CAD build for the part. Positions are in the model's coordinates, mm. Coordinates: 2 decimals unless noted, no trailing zeros. Order: outer loops, then holes, each group sorted by start corner. A loop starts at its lowest first (then second) coordinate and runs counter-clockwise, first axis right, second up. Notation, with made-up numbers: M 56.5,-14 L 103.5,-14 A30 cw 103.5,11 Z; hole C 10,9 d8. An arc over 180 degrees is marked long. Write item = value, one per line.
from build123d import *

# Parameters (mm, degrees)
SKETCH1_W           = 71.428571428
SKETCH1_H           = 3.175
SKETCH1_W_2         = 20
SKETCH1_W_3         = 18.5
BOSS_EXTRUDE1_DEPTH = 3.175


with BuildPart() as part:
    # Sketch1 → Boss-Extrude1 (new body)
    with BuildSketch(Plane.XY):
        Polygon((0, 0), (0, 132.75), (0, 252.75), (278.222222222, 252.75), (313, 252.75), (313, 228.115), (313, 132.75), (357.142857143, 132.75), (357.142857143, 129.575), (428.571428571, 129.575), (428.571428571, 132.75), (500, 132.75), (500, 0), (428.571428571, 0), (428.571428571, 3.175), (357.142857143, 3.175), (357.142857143, 0), (285.714285714, 0), (285.714285714, 3.175), (214.285714286, 3.175), (214.285714286, 0), (142.857142857, 0), (142.857142857, 3.175), (71.428571429, 3.175), (71.428571429, 0), align=None)
        with Locations((107.142857143, 131.1625)):
            Rectangle(SKETCH1_W, SKETCH1_H, mode=Mode.SUBTRACT)
        with Locations((250, 131.1625)):
            Rectangle(SKETCH1_W, SKETCH1_H, mode=Mode.SUBTRACT)
        with Locations((14, 60.0875)):
            Rectangle(SKETCH1_W_2, SKETCH1_H, mode=Mode.SUBTRACT)
        with Locations((14, 72.6625)):
            Rectangle(SKETCH1_W_2, SKETCH1_H, mode=Mode.SUBTRACT)
        with Locations((472.25, 33.2875)):
            Rectangle(SKETCH1_W_3, SKETCH1_H, mode=Mode.SUBTRACT)
        with Locations((472.25, 99.4625)):
            Rectangle(SKETCH1_W_3, SKETCH1_H, mode=Mode.SUBTRACT)
    extrude(amount=BOSS_EXTRUDE1_DEPTH)


solid = part.part
(1) Pin check, flat tips, straight feed: pin 1 Ø1.6 at (y, z) = (131, 1) entering from -X; pin 2 Ø1 at (x, z) = (472, 1) entering from +Y; pin 3 Ø1 at (x, z) = (260, 2) entering from -Y (3 decimals). Stop position of each tip, or through.
Evaluation:
pin_1 = 0
pin_2 = 132.75
pin_3 = 3.175
(2) Slice it at C-C, the plane x = 375. Write the cut outline in (y, z) (3 decimals).
Evaluation:
outline = M 3.175,0 L 129.575,0 L 129.575,3.175 L 3.175,3.175 Z
(3) Slice it at A-A, the plane x = 248.5. Write the cut outline in (y, z) (3 decimals), then the cut area to 3 significant figures.
Evaluation:
outline = M 3.175,0 L 129.575,0 L 129.575,3.175 L 3.175,3.175 Z; M 132.75,0 L 252.75,0 L 252.75,3.175 L 132.75,3.175 Z
area = 782 mm²
(4) Slice it at D-D, the plane y = 198. Write the cut outline in (x, z) (3 decimals).
Evaluation:
outline = M 0,0 L 313,0 L 313,3.175 L 0,3.175 Z
(5) Slice it at B-B, the plane z = 0.65. State how many separate pieces and enclosed holes the cut face has, then the cut area to 3 significant figures.
Evaluation:
separate_pieces = 1
enclosed_holes = 6
area = 102,000 mm²
(6) Wall check: line 1 (X direction, y = 101, z = 1.7); line 2 (Y direction, x = 278.5, z = 1.4) (3 decimals); line 3 (Y direction, x = 443.5, z = 0.95). Give the ranges that are in metal, low to high. Write a range as from..to.
Evaluation:
line_1 = 0..463, 481.5..500
line_2 = 3.175..129.575, 132.75..252.75
line_3 = 0..132.75
